Geometry check sheet. Reference: the model listing, model coordinates, mm. Face numbers are marked on the shaded views. A direction names the side the tool comes from. Give positions to 0.01 mm unless a question says otherwise; leave off trailing zeros. Order: outer loops, then holes, each group sorted by start corner. A loop starts at its lowest first (then second) coordinate and runs counter-clockwise, first axis right, second up.
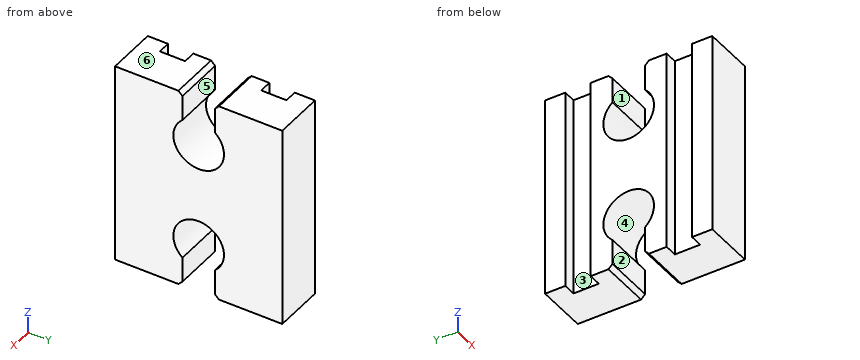
from build123d import *

# Parameters (mm, degrees)
F1_DEPTH = 50.8
F3_DEPTH = 25.4
F7_SIZE  = 1.016


with BuildPart() as f1:
    # F0 (on Top) → F1 (new body)
    with BuildSketch(Plane.XY):
        Polygon((-12.7, -15.875), (-12.7, -20.955), (0, -20.955), (0, 20.955), (-12.7, 20.955), (-12.7, 15.875), (-9.525, 15.875), (-9.525, 9.525), (-12.7, 9.525), (-12.7, -9.525), (-9.525, -9.525), (-9.525, -15.875), align=None)
    extrude(amount=F1_DEPTH)

    # F2 (on face) → F3 (cut)
    with BuildSketch(Plane.YZ):
        with BuildLine():
            Line((-4.064, 7.3128193311), (-4.064, 0))
            Line((-4.064, 0), (4.064, 0))
            Line((4.064, 0), (4.064, 7.3128193311))
            ThreePointArc((4.064, 7.3128193311), (0, 18.542), (-4.064, 7.3128193311))
        make_face()
    extrude(amount=-F3_DEPTH, mode=Mode.SUBTRACT)

    # F6: F1 across plane


with BuildPart() as f1_1:
    add(f1.part)
    add(f1.part.mirror(Plane(origin=(-5.8559647303, -12.4897385892, 25.4), x_dir=(1, 0, 0), z_dir=(0, 0, -1))), mode=Mode.INTERSECT)

    # F7
    f7_edges = [f1_1.edges().sort_by_distance(p)[0] for p in [
        (-6.35, -4.064, 50.8),
        (-6.35, 4.064, 50.8),
        (-6.35, 4.064, 0),
        (-6.35, -4.064, 0),
    ]]
    chamfer(f7_edges, length=F7_SIZE)


solid = f1_1.part
Item 1: Set-up check for the marked faces 1, 2 and 3: record each of +Z, -Z, +X, -X, +Y, -Y from which the full face is reachable in a straight line by a thin tool's end or side.
Reported:
face 1: +Z, +X, -X
face 2: -Z, +X, -X
face 3: +Z, -Z, -X
Item 2: Sectioned sample at B-B (x = -5.25). Enter the section's corners in (y, z) (3 decimals), and give its area (3 significant figures).
Reported:
outline: (-20.955, 0) - (-5.08, 0) - (-4.064, 1.016) - (-4.064, 7.313) arc R6.35 cw (long way) to (4.064, 7.313) - (4.064, 1.016) - (5.08, 0) - (20.955, 0) - (20.955, 50.8) - (5.08, 50.8) - (4.064, 49.784) - (4.064, 43.487) arc R6.35 cw (long way) to (-4.064, 43.487) - (-4.064, 49.784) - (-5.08, 50.8) - (-20.955, 50.8) - close
area: 1,770 mm2
Item 3: Sectioned sample at D-D (y = -11.5). Enter the section's corners in (x, z) (3 decimals), and give its area (3 significant figures).
Reported:
outline: (-9.525, 0) - (0, 0) - (0, 50.8) - (-9.525, 50.8) - close
area: 484 mm2
Item 4: Scan lines: L1, parallel to Y at x = -4, z = 49 (3 decimals); L2, parallel to Y at x = -9.75, z = 4 (3 decimals); L3, parallel to Y at x = -10.5, z = 18 (3 decimals). Record each from-to range of solid material in increasing order.
Reported:
L1: y = -20.955 to -4.064, 4.064 to 20.955
L2: y = -20.955 to -15.875, -9.525 to -4.064, 4.064 to 9.525, 15.875 to 20.955
L3: y = -20.955 to -15.875, -9.525 to -2.567, 2.567 to 9.525, 15.875 to 20.955
Item 5: Gauge pin test, flat ends, axial feed: pin 1 (5 mm diameter, centred on y = -14, z = 27.5, fed in from -X); pin 2 (3 mm diameter, centred on y = 13.5, z = 31.5, fed in from -X) (3 decimals). Record the tip position at first contact, or that the pin passes through.
Reported:
pin 1: stops at x = -12.7
pin 2: stops at x = -9.525
Item 6: Sectioned sample at A-A (z = 22). Enter the section's corners in (x, y) (3 decimals).
Reported:
outline: (-12.7, -20.955) - (0, -20.955) - (0, 20.955) - (-12.7, 20.955) - (-12.7, 15.875) - (-9.525, 15.875) - (-9.525, 9.525) - (-12.7, 9.525) - (-12.7, -9.525) - (-9.525, -9.525) - (-9.525, -15.875) - (-12.7, -15.875) - close
Item 7: Draft check along Z on the marked faces 4, 5 and 6. Enter one of: released by +Z, released by -Z, zero draft, split by the parting line, or undercut.
Reported:
face 4: undercut
face 5: zero draft
face 6: released by +Z
Item 8: Sectioned sample at C-C (z = 33.5). Enter the section's corners in (x, y) (3 decimals).
Reported:
outline: (-12.7, -20.955) - (0, -20.955) - (0, -3.772) - (-12.7, -3.772) - (-12.7, -9.525) - (-9.525, -9.525) - (-9.525, -15.875) - (-12.7, -15.875) - close; (-12.7, 3.772) - (0, 3.772) - (0, 20.955) - (-12.7, 20.955) - (-12.7, 15.875) - (-9.525, 15.875) - (-9.525, 9.525) - (-12.7, 9.525) - close
